Part model, mm, in its own coordinate system. A direction names the side the tool comes from. Round coordinates to 2 decimals unless told otherwise and drop trailing zeros. Order: outer loops, then holes, each group sorted by start corner. A loop starts at its lowest first (then second) coordinate and runs counter-clockwise, first axis right, second up. Notation, with made-up numbers: (80.5, 20.5) -> (93.5, 20.5) arc R15 cw to (93.5, 33.5) -> close; hole circle Ø3 at (19, -24.75). An arc over 180 degrees is marked (long way). Answer as a JSON object with one key per item and string values. Group by question number.
```python
from build123d import *

# Parameters (mm, degrees)
SKETCH_W        = 114
SKETCH_H        = 47
PAD_DEPTH       = 24.5
THICKNESS_T     = -2
SKETCH001_W     = 114
SKETCH001_H     = 1.1
POCKET_DEPTH    = 1.5
SKETCH002_W     = 1.1
SKETCH002_H     = 47
POCKET001_DEPTH = 1.5
SKETCH003_W     = 10
SKETCH003_H     = 23
PAD001_DEPTH    = 10
SKETCH004_W     = 10
SKETCH004_H     = 23
PAD002_DEPTH    = 10
SKETCH005_R     = 1.25
POCKET002_DEPTH = 23
SKETCH006_R     = 0.5
POCKET003_DEPTH = 2
SKETCH007_W     = 9
SKETCH007_H     = 5
PAD003_DEPTH    = 6
SKETCH009_R     = 1.5
POCKET004_DEPTH = 5
FILLET_R        = 3
FILLET001_R     = 3
FILLET002_R     = 3


with BuildPart() as part:
    # Sketch → Pad (new body)
    with BuildSketch(Plane.XY):
        Rectangle(SKETCH_W, SKETCH_H)
    extrude(amount=PAD_DEPTH)

    # Thickness
    thickness_openings = [part.faces().sort_by_distance(p)[0] for p in [
        (0, 0, 24.5),
    ]]
    offset(amount=THICKNESS_T, openings=thickness_openings)

    # Sketch001 (on Face6 of Thickness) → Pocket (cut)
    with BuildSketch(Plane.XY.offset(24.5)):
        with Locations((0, -22.95)):
            Rectangle(SKETCH001_W, SKETCH001_H)
        with Locations((0, 22.95)):
            Rectangle(SKETCH001_W, SKETCH001_H)
    extrude(amount=-POCKET_DEPTH, mode=Mode.SUBTRACT)

    # Sketch002 (on Face6 of Pocket) → Pocket001 (cut)
    with BuildSketch(Plane.XY.offset(24.5)):
        with Locations((56.45, 0)):
            Rectangle(SKETCH002_W, SKETCH002_H)
        with Locations((-56.45, 0)):
            Rectangle(SKETCH002_W, SKETCH002_H)
    extrude(amount=-POCKET001_DEPTH, mode=Mode.SUBTRACT)

    # Sketch003 (on Face4 of Pocket001) → Pad001 (join)
    with BuildSketch(Plane(origin=(0, 23.5, 0), x_dir=(-1, 0, 0), z_dir=(0, 1, 0))):
        with Locations((-52, 11.5)):
            Rectangle(SKETCH003_W, SKETCH003_H)
        with Locations((52, 11.5)):
            Rectangle(SKETCH003_W, SKETCH003_H)
    extrude(amount=PAD001_DEPTH)

    # Sketch004 (on Face1 of Pad001) → Pad002 (join)
    with BuildSketch(Plane.XZ.offset(23.5)):
        with Locations((-52, 11.5)):
            Rectangle(SKETCH004_W, SKETCH004_H)
        with Locations((52, 11.5)):
            Rectangle(SKETCH004_W, SKETCH004_H)
    extrude(amount=PAD002_DEPTH)

    # Sketch005 (on Face12 of Pad002) → Pocket002 (cut)
    with BuildSketch(Plane.XY.offset(23)):
        with Locations((-52, 28.5)):
            Circle(SKETCH005_R)
        with Locations((52, 28.5)):
            Circle(SKETCH005_R)
        with Locations((52, -28.5)):
            Circle(SKETCH005_R)
        with Locations((-52, -28.5)):
            Circle(SKETCH005_R)
    extrude(amount=-POCKET002_DEPTH, mode=Mode.SUBTRACT)

    # Sketch006 (on Face12 of Pocket002) → Pocket003 (cut)
    with BuildSketch(Plane.YZ.offset(57)):
        with Locations((7.5, 10.5)):
            Circle(SKETCH006_R)
        with Locations((7.5, 15.5)):
            Circle(SKETCH006_R)
        with Locations((-7.5, 10.5)):
            Circle(SKETCH006_R)
        with Locations((-7.5, 15.5)):
            Circle(SKETCH006_R)
    extrude(amount=-POCKET003_DEPTH, mode=Mode.SUBTRACT)

    # Sketch007 (on Face4 of Pocket003) → Pad003 (join)
    with BuildSketch(Plane(origin=(-57, 0, 0), x_dir=(0, -1, 0), z_dir=(-1, 0, 0))):
        with Locations((0, 11.5)):
            Rectangle(SKETCH007_W, SKETCH007_H)
    extrude(amount=PAD003_DEPTH)

    # Sketch009 (on Face22 of Pad003) → Pocket004 (cut)
    with BuildSketch(Plane.XY.offset(14)):
        with Locations((-58.5, 0)):
            Circle(SKETCH009_R)
    extrude(amount=-POCKET004_DEPTH, mode=Mode.SUBTRACT)

    # Fillet
    fillet_edges = [part.edges().sort_by_distance(p)[0] for p in [
        (-57, -33.5, 11.5),
        (-47, -33.5, 11.5),
        (47, -33.5, 11.5),
        (57, -33.5, 11.5),
    ]]
    fillet(fillet_edges, radius=FILLET_R)

    # Fillet001
    fillet001_edges = [part.edges().sort_by_distance(p)[0] for p in [
        (-63, -4.5, 11.5),
        (-63, 4.5, 11.5),
    ]]
    fillet(fillet001_edges, radius=FILLET001_R)

    # Fillet002
    fillet002_edges = [part.edges().sort_by_distance(p)[0] for p in [
        (57, 33.5, 11.5),
        (47, 33.5, 11.5),
        (-47, 33.5, 11.5),
        (-57, 33.5, 11.5),
    ]]
    fillet(fillet002_edges, radius=FILLET002_R)


solid = part.part
```
Q1. Band-saw the part on B-B (x = -52). List the corners of the cut face in (y, z).
Q2. Band-saw the part on A-A (y = -28.5). List the corners of the cut face in (x, z), plus the area to 3 significant figures.
Q3. Drop flat-ended pins along their axis: pin 1 Ø3 at (x, y) = (-60, -1.5) entering from +Z; pin 2 Ø2 at (y, z) = (25.5, 10.5) entering from -X; pin 3 Ø7 at (x, z) = (-15.5, 10.5) entering from -Y. Give the stop position or say it passes through.
Q4. Two-plate mould, pull along X, no slides. Class faces 1 (the cylindrical face through (-57, 0, 12)), 2 (the flat face through (-52, 33.5, 12)): +X half, -X half, draft (parallel to the pull), parting line (faces both ways), or undercut.
Q5. Band-saw the part on D-D (x = -33). List the corners of the cut face in (y, z), plus the area to 3 significant figures.
Q6. Wall check: line 1 (Y direction, x = 52, z = 11.5); line 2 (Z direction, x = 56.6, y = -7.5); line 3 (X direction, y = -19.5, z = 22.25). Give the ranges that are in metal, low to high. Write a range as [from, to].
Q7. Which spindle directions (+Z, -Z, +X, -X, +Y, -Y) get a long thin tool onto all of the face, cutting with end or side? Do faces 3 (the cylindrical face through (-47.9, -32.64, 11.66)), 4 (the flat face through (-1, 21.5, 13)), 5 (the flat face through (-58, -4.5, 11)). Say none if no direction does.
Q8. Band-saw the part on C-C (y = -11.5). List the corners of the cut face in (x, z), plus the area to 3 significant figures.
Completed:
{
 "1": {"outline": "(-33.5, 0) -> (-29.75, 0) -> (-29.75, 23) -> (-33.5, 23) -> close; (-27.25, 0) -> (27.25, 0) -> (27.25, 23) -> (22.4, 23) -> (22.4, 24.5) -> (21.5, 24.5) -> (21.5, 2) -> (-21.5, 2) -> (-21.5, 24.5) -> (-22.4, 24.5) -> (-22.4, 23) -> (-27.25, 23) -> close; (29.75, 0) -> (33.5, 0) -> (33.5, 23) -> (29.75, 23) -> close"},
 "2": {"outline": "(-57, 0) -> (-53.25, 0) -> (-53.25, 23) -> (-57, 23) -> close; (-50.75, 0) -> (-47, 0) -> (-47, 23) -> (-50.75, 23) -> close; (47, 0) -> (50.75, 0) -> (50.75, 23) -> (47, 23) -> close; (53.25, 0) -> (57, 0) -> (57, 23) -> (53.25, 23) -> close", "area": "345 mm2"},
 "3": {"pin 1": "z = 14", "pin 2": "x = -57", "pin 3": "y = -23.5"},
 "4": {"face 1": "undercut", "face 2": "draft"},
 "5": {"outline": "(-23.5, 0) -> (23.5, 0) -> (23.5, 23) -> (22.4, 23) -> (22.4, 24.5) -> (21.5, 24.5) -> (21.5, 2) -> (-21.5, 2) -> (-21.5, 24.5) -> (-22.4, 24.5) -> (-22.4, 23) -> (-23.5, 23) -> close", "area": "181 mm2"},
 "6": {"line 1": "[-33.5, -29.75], [-27.25, -21.5], [21.5, 27.25], [29.75, 33.5]", "line 2": "[0, 10], [11, 15], [16, 23]", "line 3": "[-57, -55], [55, 57]"},
 "7": {"face 3": "+Z, -Z, -Y", "face 4": "+Z", "face 5": "+Z, -Z, -X, -Y"},
 "8": {"outline": "(-57, 0) -> (57, 0) -> (57, 23) -> (55.9, 23) -> (55.9, 24.5) -> (55, 24.5) -> (55, 2) -> (-55, 2) -> (-55, 24.5) -> (-55.9, 24.5) -> (-55.9, 23) -> (-57, 23) -> close", "area": "315 mm2"}
}
